Check sheet for the drawn part. Datum: minimum x, y, z corner. Units: mm. Give positions to 0.01 mm unless a question says otherwise; leave off trailing zeros. Write each loop counter-clockwise with the first axis right and the second up, starting at its lowest first coordinate (ties: lowest second). Pieces come first, ordered by that corner, then holes. Notation, with made-up numbers: (75.25, 54) - (121.25, 54) arc R18 ccw to (121.25, 74) - close; hole circle Ø11 at (1, 82.25). An arc over 180 degrees is marked (long way). Use a Markdown table: item, result.
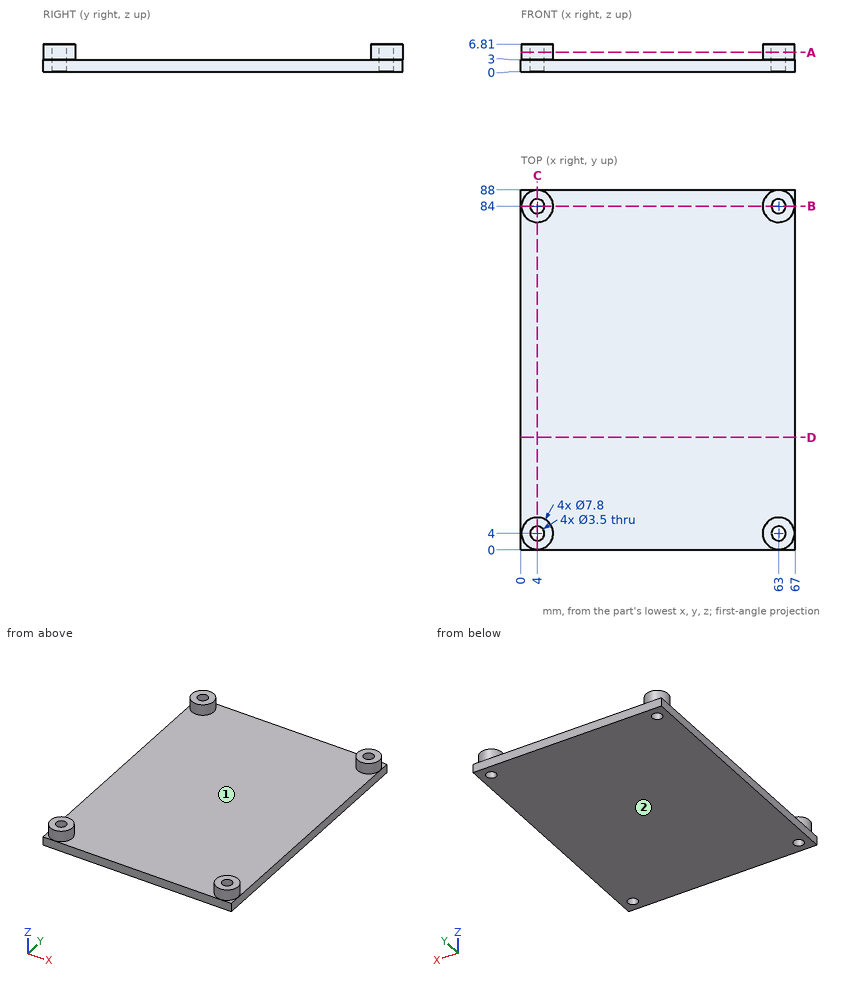
1) Material ranges on L1, parallel to Y at x = 4, z = 3.75; L2, parallel to X at y = 4, z = 2; L3, parallel to Y at x = 63, z = 1.5, recorded low to high. Write a range as from..to.
Working result:
| item | result |
|---|---|
| L1 | y = 0.1..2.25, 5.75..7.9, 80.1..82.25, 85.75..87.9 |
| L2 | x = 0..2.25, 5.75..61.25, 64.75..67 |
| L3 | y = 0..2.25, 5.75..82.25, 85.75..88 |
2) Section check B-B on y = 84. Record the boundary of the cut face in (x, z), then the cut area to 3 significant figures.
Working result:
| item | result |
|---|---|
| outline | (0, 0) - (2.25, 0) - (2.25, 6.81) - (0.1, 6.81) - (0.1, 3) - (0, 3) - close; (5.75, 0) - (61.25, 0) - (61.25, 6.81) - (59.1, 6.81) - (59.1, 3) - (7.9, 3) - (7.9, 6.81) - (5.75, 6.81) - close; (64.75, 0) - (67, 0) - (67, 3) - (66.9, 3) - (66.9, 6.81) - (64.75, 6.81) - close |
| area | 213 mm² |
3) Section check D-D on y = 27.5. Record the boundary of the cut face in (x, z), then the cut area to 3 significant figures.
Working result:
| item | result |
|---|---|
| outline | (0, 0) - (67, 0) - (67, 3) - (0, 3) - close |
| area | 201 mm² |
4) Section check A-A on z = 4.75. Record the boundary of the cut face in (x, y), then the cut area to 3 significant figures.
Working result:
| item | result |
|---|---|
| outline | circle Ø7.8 at (4, 4); circle Ø7.8 at (4, 84); circle Ø7.8 at (63, 4); circle Ø7.8 at (63, 84); hole circle Ø3.5 at (4, 4); hole circle Ø3.5 at (4, 84); hole circle Ø3.5 at (63, 4); hole circle Ø3.5 at (63, 84) |
| area | 153 mm² |
5) Depth check by flat-ended pin: P1, Ø20, axis at x = 49, y = 56.5, coming from the +Z side. Enter the tip coordinate at first touch or a pass-through.
Working result:
| item | result |
|---|---|
| P1 | stops at z = 3 |
6) Section check C-C on x = 4. Record the boundary of the cut face in (y, z), then the cut area to 3 significant figures.
Working result:
| item | result |
|---|---|
| outline | (0, 0) - (2.25, 0) - (2.25, 6.81) - (0.1, 6.81) - (0.1, 3) - (0, 3) - close; (5.75, 0) - (82.25, 0) - (82.25, 6.81) - (80.1, 6.81) - (80.1, 3) - (7.9, 3) - (7.9, 6.81) - (5.75, 6.81) - close; (85.75, 0) - (88, 0) - (88, 3) - (87.9, 3) - (87.9, 6.81) - (85.75, 6.81) - close |
| area | 276 mm² |
7) Mould release check, pull along Y, two halves, no side actions. Record for the marked faces 1 and 2: pulls with the +Y half, pulls with the -Y half, needs draft (parallel to the pull), parting line crosses it, or undercut.
Working result:
| item | result |
|---|---|
| face 1 | undercut |
| face 2 | needs draft |
